Could you check a few things on this model? Use its own coordinates, in mm. Face numbers are marked on the shaded views. A direction names the side the tool comes from. Round coordinates to 2 decimals unless told otherwise and drop trailing zeros. Write each loop counter-clockwise with the first axis right and the second up, starting at its lowest first coordinate (ties: lowest second). Pieces come first, ordered by that corner, then holes. Notation, with made-up numbers: M 40,46.5 L 66,46.5 A14 ccw 66,59.5 Z; hole C 88.25,-21.5 d6. An arc over 180 degrees is marked long. One line per item, written item: value. Start each with the question number.
(1) I want a section at B-B on x = 700. Please give me the cut outline in (y, z), and give its area (3 significant figures).
(2) Which directions (+Z, -Z, +X, -X, +Y, -Y) give clear straight access to the entire face, cutting with the end or side of a thin tool? Please do the marked faces 1 and 2.
(3) I'm going to push flat-ended pins straight in: pin 1 Ø8 at (x, y) = (-253.5, -459) entering from -Z; pin 2 Ø2 at (x, z) = (70, 388.5) entering from +Y; pin 3 Ø6 at (x, y) = (-623, -138) entering from +Z. Where does each tip first touch, or does it pass through?
(4) I want a section at D-D on z = -95. Please give me the cut outline in (x, y), and give its area (3 significant figures).
(5) I want a section at C-C on y = -151.5. Please give me the cut outline in (x, z).
(6) If I drill on L1, parallel to Z at x = 520, y = -143.5; L2, parallel to X at y = -6, z = 0; L3, parallel to X at y = -155, z = -440, over which ranges is the centre line in solid material (lowest first)?
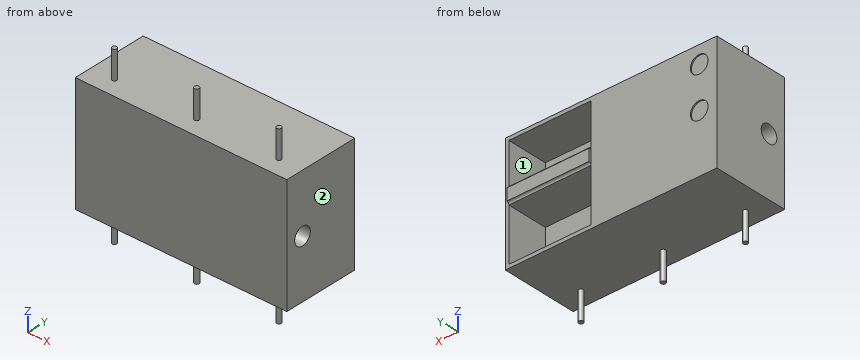
```python
from build123d import *

# Parameters (mm, degrees)
SKIZZE1_W                            = 1800
SKIZZE1_H                            = 1000
AUFSATZ_LINEAR_AUSTRAGEN1_DEPTH      = 650
AUFSATZ_LINEAR_AUSTRAGEN2_DEPTH      = 740
AUFSATZ_LINEAR_AUSTRAGEN2_DEPTH_BACK = 740
SKIZZE2_R                            = 20
SKIZZE3_W                            = 700
SKIZZE3_H                            = 450
SKIZZE3_H_2                          = 350
SCHNITT_LINEAR_AUSTRAGEN1_DEPTH      = 350
SKIZZE4_W                            = 700
SKIZZE4_H                            = 140
AUFSATZ_LINEAR_AUSTRAGEN3_DEPTH      = 20
SKIZZE5_R                            = 20
SCHNITT_LINEAR_AUSTRAGEN2_DEPTH      = 700
SKIZZE6_R                            = 75
SCHNITT_LINEAR_AUSTRAGEN3_DEPTH      = 1800
SKIZZE7_R                            = 75
SCHNITT_LINEAR_AUSTRAGEN4_DEPTH      = 10
SKIZZE8_R                            = 75
SCHNITT_LINEAR_AUSTRAGEN5_DEPTH      = 10


with BuildPart() as part:
    # Skizze1 → Aufsatz-Linear austragen1 (new body)
    with BuildSketch(Plane(origin=(0, 0, 0), x_dir=(1, 0, 0), z_dir=(0, 1, 0))):
        Rectangle(SKIZZE1_W, SKIZZE1_H)
    extrude(amount=-AUFSATZ_LINEAR_AUSTRAGEN1_DEPTH)

    # Skizze2 → Aufsatz-Linear austragen2 (add, two sides: drawn at the far end of the back side and taken through both)
    with BuildSketch(Plane.XY.offset(-AUFSATZ_LINEAR_AUSTRAGEN2_DEPTH_BACK)):
        with Locations((0, -500)):
            Circle(SKIZZE2_R)
        with Locations((-700, -500)):
            Circle(SKIZZE2_R)
        with Locations(Location((700, -500, 0), (0, 0, 180))):
            Circle(SKIZZE2_R)
    extrude(amount=AUFSATZ_LINEAR_AUSTRAGEN2_DEPTH + AUFSATZ_LINEAR_AUSTRAGEN2_DEPTH_BACK)

    # Skizze3 → Schnitt-Linear austragen1 (cut)
    with BuildSketch(Plane(origin=(0, 0, 0), x_dir=(1, 0, 0), z_dir=(0, 1, 0))):
        with Locations((520, 245)):
            Rectangle(SKIZZE3_W, SKIZZE3_H)
        with Locations((520, -295)):
            Rectangle(SKIZZE3_W, SKIZZE3_H_2)
    extrude(amount=-SCHNITT_LINEAR_AUSTRAGEN1_DEPTH, mode=Mode.SUBTRACT)

    # Skizze4 → Aufsatz-Linear austragen3 (add)
    with BuildSketch(Plane(origin=(0, 0, 0), x_dir=(1, 0, 0), z_dir=(0, 1, 0))):
        with Locations((520, -50)):
            Rectangle(SKIZZE4_W, SKIZZE4_H)
    extrude(amount=AUFSATZ_LINEAR_AUSTRAGEN3_DEPTH)

    # Skizze5 → Schnitt-Linear austragen2 (cut)
    with BuildSketch(Plane(origin=(870, 0, 0), x_dir=(0, 0, -1), z_dir=(1, 0, 0))):
        with Locations((-120, 20)):
            Circle(SKIZZE5_R)
        with Locations((20, 20)):
            Circle(SKIZZE5_R)
    extrude(amount=-SCHNITT_LINEAR_AUSTRAGEN2_DEPTH, mode=Mode.SUBTRACT)

    # Skizze6 → Schnitt-Linear austragen3 (cut)
    with BuildSketch(Plane(origin=(900, 0, 0), x_dir=(0, 0, -1), z_dir=(1, 0, 0))):
        with Locations((0, -500)):
            Circle(SKIZZE6_R)
    extrude(amount=-SCHNITT_LINEAR_AUSTRAGEN3_DEPTH, mode=Mode.SUBTRACT)

    # Skizze7 → Schnitt-Linear austragen4 (cut)
    with BuildSketch(Plane(origin=(0, 0, 0), x_dir=(1, 0, 0), z_dir=(0, 1, 0))):
        with Locations(Location((-750, -350, 0), (0, 0, 270))):
            Circle(SKIZZE7_R)
    extrude(amount=-SCHNITT_LINEAR_AUSTRAGEN4_DEPTH, mode=Mode.SUBTRACT)

    # Skizze8 → Schnitt-Linear austragen5 (cut)
    with BuildSketch(Plane(origin=(0, 0, 0), x_dir=(1, 0, 0), z_dir=(0, 1, 0))):
        with Locations(Location((-750, 0, 0), (0, 0, 270))):
            Circle(SKIZZE8_R)
    extrude(amount=-SCHNITT_LINEAR_AUSTRAGEN5_DEPTH, mode=Mode.SUBTRACT)


solid = part.part
```
Found:
1. outline: M -650,-500 L -520,-500 L -520,-740 L -480,-740 L -480,-500 L 0,-500 L 0,-470 L -350,-470 L -350,-20 L 0,-20 A20 cw 20,0 L 20,100 A20 cw 0,120 L -350,120 L -350,470 L 0,470 L 0,500 L -480,500 L -480,740 L -520,740 L -520,500 L -650,500 Z; hole C -500,0 d150
1. area: 374,000 mm²
2. face 1: +Y
2. face 2: +Z, -Z, +X, +Y, -Y
3. pin 1: stops at z = -500
3. pin 2: stops at y = 0
3. pin 3: stops at z = 500
4. outline: M -900,-650 L 900,-650 L 900,0 L 870,0 L 870,-350 L 170,-350 L 170,0 L -900,0 Z
4. area: 925,000 mm²
5. outline: M -900,-500 L 900,-500 L 900,500 L -900,500 Z; hole M 170,-470 L 870,-470 L 870,-20 L 170,-20 Z; hole M 170,120 L 870,120 L 870,470 L 170,470 Z
6. L1: z = -500 to -470, -20 to 120, 470 to 500
6. L2: x = -900 to -825, -675 to 900
6. L3: x = -900 to 170, 870 to 900
